Here's the drawing with two shaded views (mm, measured from the low corner). I have some questions. Give positions to 0.01 mm unless a question says otherwise; leave off trailing zeros. Write each loop counter-clockwise with the first axis right and the second up, starting at its lowest first coordinate (ties: lowest second). Pieces come first, ordered by that corner, then holes. Notation, with made-up numbers: (21, -20) -> (25, -20) arc R9 cw to (25, -11) -> close; hole circle Ø6 at (-9, -7). An arc over 180 degrees is marked (long way). One line per item, written item: value.
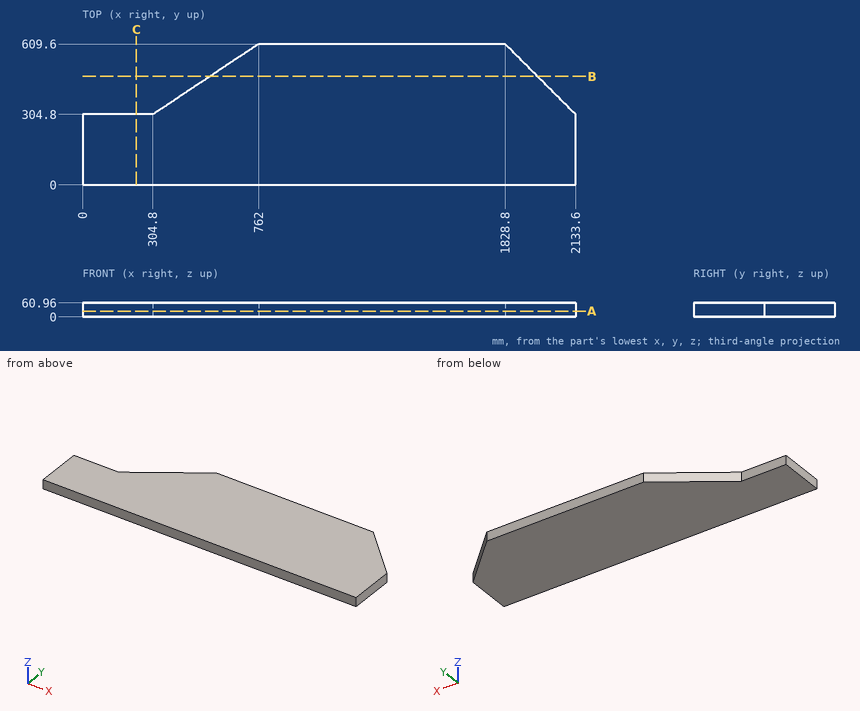
1) I need wall thicknesses on L1, parallel to Y at x = 109.5, z = 50.5; L2, parallel to Y at x = 626.5, z = 11; L3, parallel to X at y = 341.5, z = 43. Which ranges of each line are inside material? Lowest first, please.
Answer list:
L1: y = 0 to 304.8
L2: y = 0 to 519.27
L3: x = 359.85 to 2096.9
2) If we section it at C-C (x = 233.5): Write out the boundary of the cut face in (y, z), and give its area (3 significant figures).
Answer list:
outline: (0, 0) -> (304.8, 0) -> (304.8, 60.96) -> (0, 60.96) -> close
area: 18,600 mm^2
3) If we section it at B-B (y = 469.5): Write out the boundary of the cut face in (x, z), and give its area (3 significant figures).
Answer list:
outline: (551.85, 0) -> (1968.9, 0) -> (1968.9, 60.96) -> (551.85, 60.96) -> close
area: 86,400 mm^2
4) Will these pins go through, and if not, where does the flat tip stop? pin 1 (8 mm diameter, centred on y = 311, z = 31, fed in from -X); pin 2 (5 mm diameter, centred on x = 1903, z = 8, fed in from +Y); pin 3 (12 mm diameter, centred on y = 353, z = 20, fed in from +X).
Answer list:
pin 1: stops at x = 308.1
pin 2: stops at y = 537.9
pin 3: stops at x = 2091.4
5) If we section it at A-A (z = 25): Write out the boundary of the cut face in (x, y).
Answer list:
outline: (0, 0) -> (2133.6, 0) -> (2133.6, 304.8) -> (1828.8, 609.6) -> (762, 609.6) -> (304.8, 304.8) -> (0, 304.8) -> close
